Source: three-view drawing plus pictorial views. Frame: mm from the lowest corner of the part. A direction names the side the tool comes from. Give positions to 0.01 mm unless a question says otherwise; leave off trailing zeros. Order: outer loops, then holes, each group sorted by start corner. A loop starts at its lowest first (then second) coordinate and runs counter-clockwise, first axis right, second up. Notation, with made-up numbers: M -4.75,19.5 L 32.25,19.5 A11 ccw 32.25,34.5 Z; hole C 37,25 d6. An arc over 180 degrees is marked long. Use CSV: the item, a comma, the result in double quotes. Start each with the question number.
1. Section query B-B, the plane x = 7.5. Return the cut outline in (y, z) (3 decimals), plus the area to 4 significant figures.
2. Reachability of the marked faces 5, 6 and 7 from +Z, -Z, +X, -X, +Y, -Y: full face, straight path, thin tool, end or side. Return the list, or none.
3. Section query D-D, the plane y = 1.1. Return the cut outline in (x, z), plus the area to 3 significant figures.
4. Pin query (flat end, axial travel): P1, Ø1.1, axis at y = 1, z = 13.5, coming from the -X side; P2, Ø0.6, axis at x = 7, y = 2, coming from the +Z side; P3, Ø2, axis at x = 8, z = 13, coming from the +Y side. Return the tip coordinate at first contact, or that it passes through.
5. Mould query, pull axis X, two halves, no side actions, for the marked faces 1, 2, 3 and 4. Classes: released by +X, released by -X, zero draft, split by the parting line, or undercut.
6. Section query C-C, the plane z = 7.5. Return the cut outline in (x, y) (3 decimals).
7. Section query A-A, the plane x = 12.25. Return the cut outline in (y, z).
8. Line query: line 1 along X through (y, z) = (0.95, 12.25); line 2 along X through (y, z) = (1.05, 2.75); line 3 along Z through (x, y) = (3, 0.7). Output: solid intervals per line, ascending. Write a range as [from, to].
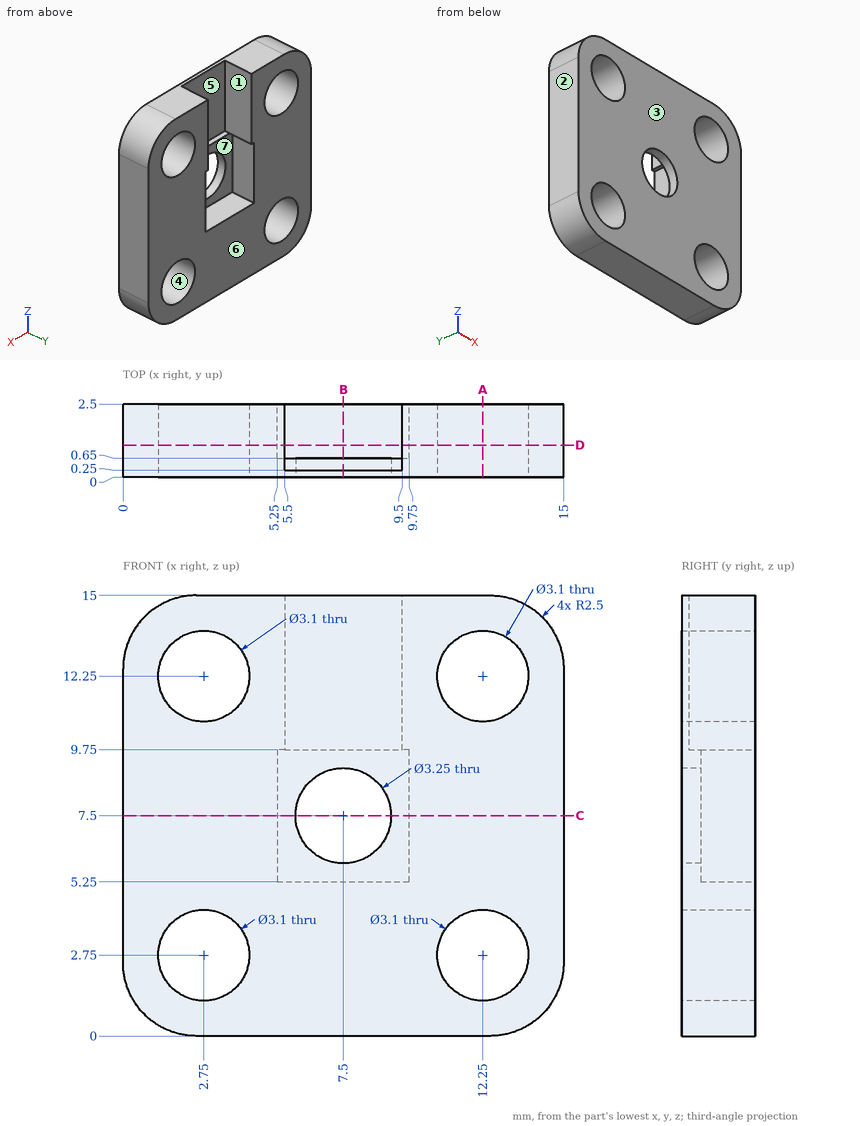
Result set:
1,outline,"M 0,0 L 2.5,0 L 2.5,5.25 L 0.65,5.25 L 0.65,5.875 L 0,5.875 Z; M 0,9.125 L 0.65,9.125 L 0.65,9.75 L 0.25,9.75 L 0.25,15 L 0,15 Z"
1,area,"15.25 mm2"
2,face 5,"+Z, +Y"
2,face 6,"+Z, -Z, +X, -X, +Y"
2,face 7,"+Y"
3,outline,"M 0,2.5 A2.5 ccw 2.5,0 L 12.5,0 A2.5 ccw 15,2.5 L 15,12.5 A2.5 ccw 12.5,15 L 9.5,15 L 9.5,9.75 L 9.75,9.75 L 9.75,5.25 L 5.25,5.25 L 5.25,9.75 L 5.5,9.75 L 5.5,15 L 2.5,15 A2.5 ccw 0,12.5 Z; hole C 2.75,2.75 d3.1; hole C 2.75,12.25 d3.1; hole C 12.25,2.75 d3.1; hole C 12.25,12.25 d3.1"
3,area,"148 mm2"
4,P1,"x = 0.04"
4,P2,"z = 5.25"
4,P3,"y = 0.25"
5,face 1,"undercut"
5,face 2,"released by -X"
5,face 3,"zero draft"
5,face 4,"undercut"
6,outline,"M 0,0 L 5.875,0 L 5.875,0.65 L 5.25,0.65 L 5.25,2.5 L 0,2.5 Z; M 9.125,0 L 15,0 L 15,2.5 L 9.75,2.5 L 9.75,0.65 L 9.125,0.65 Z"
7,outline,"M 0,0 L 2.5,0 L 2.5,1.2 L 0,1.2 Z; M 0,4.3 L 2.5,4.3 L 2.5,10.7 L 0,10.7 Z; M 0,13.8 L 2.5,13.8 L 2.5,15 L 0,15 Z"
8,line 1,"[0, 1.2], [4.3, 5.5], [9.5, 10.7], [13.8, 15]"
8,line 2,"[0, 1.2], [4.3, 10.7], [13.8, 15]"
8,line 3,"[0, 1.22], [4.28, 10.72], [13.78, 15]"
